Job drawing, mm, ordinate dimensions from the low corner. One solid piece. A direction names the side the tool comes from. Round coordinates to 2 decimals unless told otherwise and drop trailing zeros. Order: outer loops, then holes, each group sorted by start corner. A loop starts at its lowest first (then second) coordinate and runs counter-clockwise, first axis right, second up. Notation, with made-up numbers: (77, 32.5) -> (127, 32.5) arc R16 ccw to (127, 59.5) -> close; hole circle Ø7 at (4.25, 28.25). An arc over 180 degrees is marked (long way). Write item = value, one per line.
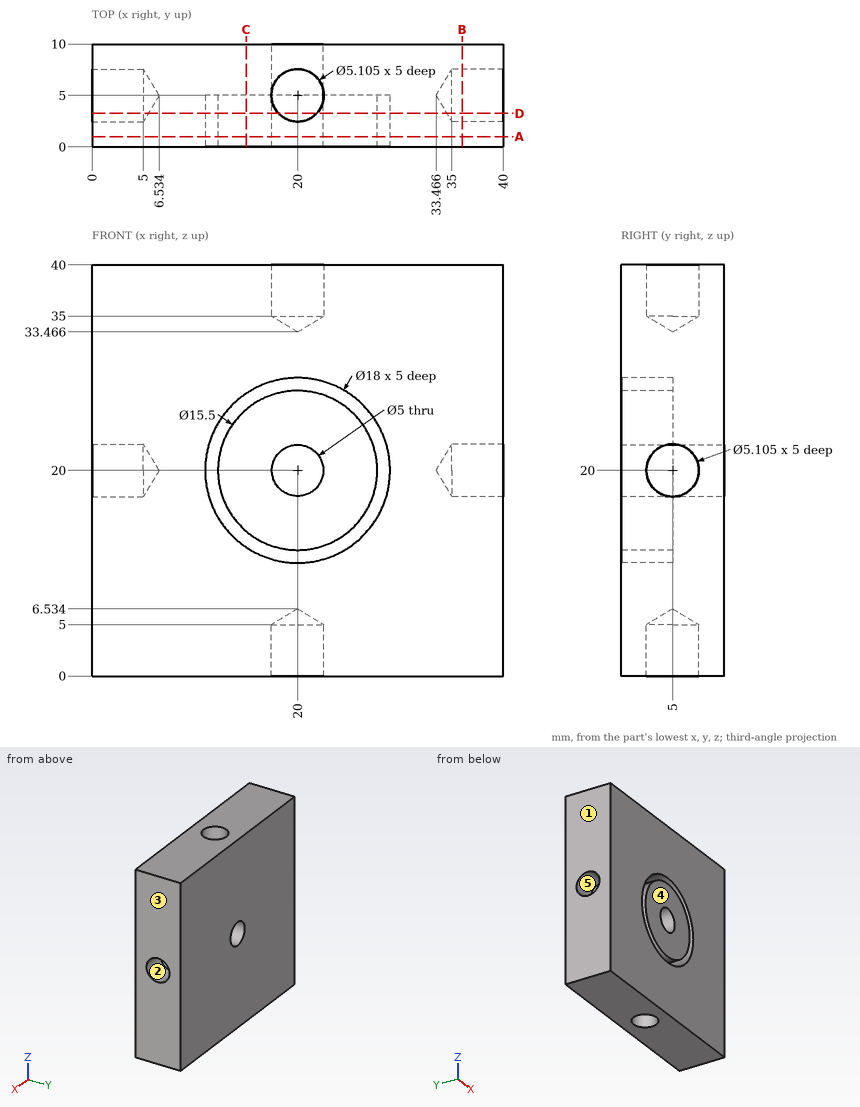
Q1. Mould opens along Y. For the marked faces 3, 4 and 5 say: released by +Y, released by -Y, zero draft, split by the parting line, or undercut.
Check values:
face_3 = zero draft
face_4 = released by -Y
face_5 = undercut
Q2. Flat gauge pins, fed straight in: pin 1 (3 mm diameter, centred on x = 20, y = 5, fed in from -Z); pin 2 (4.5 mm diameter, centred on y = 5, z = 20, fed in from -X); pin 3 (3 mm diameter, centred on x = 20, z = 20, fed in from +Y) (3 decimals); pin 4 (4 mm diameter, centred on y = 5, z = 20, fed in from +X). Where does each tip first touch, or does it go through?
Check values:
pin_1 = 5.63
pin_2 = 5.18
pin_3 = through
pin_4 = 34.67
Q3. Which spindle directions (+Z, -Z, +X, -X, +Y, -Y) get a long thin tool onto all of the face, cutting with end or side? Do the marked faces 1 and 2. Say none if no direction does.
Check values:
face_1 = +Z, -Z, -X, +Y, -Y
face_2 = +X
Q4. Cut at A-A, the plane y = 1. List the corners of the cut face in (x, z), and give its area (3 significant figures).
Check values:
outline = (0, 0) -> (40, 0) -> (40, 40) -> (0, 40) -> close; circle Ø15.5 at (20, 20); hole circle Ø18 at (20, 20); hole circle Ø5 at (20, 20)
area = 1,510 mm²
Q5. Cut at D-D, the plane y = 3.25. Give the number of separate pieces and of enclosed holes in the cut face, and give its area (3 significant figures).
Check values:
separate_pieces = 2
enclosed_holes = 2
area = 1,440 mm²
Q6. Cut at B-B, the plane x = 36. List the corners of the cut face in (y, z) (1 decimal).
Check values:
outline = (0, 0) -> (10, 0) -> (10, 40) -> (0, 40) -> close; hole circle Ø5.1 at (5, 20)
Q7. Probe probe 1 along X at (y, z) = (5, 36.7); probe 2 along Y at (x, z) = (2, 20); probe 3 along Z at (x, y) = (19, 2.75) (1 decimal). List the from-to ranges inside material, lowest first.
Check values:
probe_1 = 0 to 17.45, 22.55 to 40
probe_2 = 0 to 2.45, 7.55 to 10
probe_3 = 5.1 to 11.1, 12.3 to 17.7, 22.3 to 27.7, 28.9 to 34.9
Q8. Cut at C-C, the plane x = 15. List the corners of the cut face in (y, z), and give its area (3 significant figures).
Check values:
outline = (0, 0) -> (10, 0) -> (10, 40) -> (0, 40) -> (0, 27.48) -> (5, 27.48) -> (5, 25.92) -> (0, 25.92) -> (0, 14.08) -> (5, 14.08) -> (5, 12.52) -> (0, 12.52) -> close
area = 384 mm²
